Design review of the part built by this model. Coordinates are the model's own, in mm. A direction names the side the tool comes from. Coordinates: 2 decimals unless noted, no trailing zeros. Write each loop counter-clockwise with the first axis right and the second up, starting at its lowest first coordinate (ties: lowest second). Pieces come first, ordered by that corner, then holes. Notation, with made-up numbers: (-20, 13.25) - (16, 13.25) arc R31 cw to (16, 52.25) - close; hole circle Ø6 at (75.5, 65.25). An arc over 180 degrees is marked (long way). Answer as a JSON object with one key per item and string values.
```python
from build123d import *

# Parameters (mm, degrees)
SKETCH2_W               = 52
SKETCH2_H               = 58.5
SKETCH2_R               = 1.7
SKETCH2_R_2             = 2.65
BOSS_EXTRUDE1_DEPTH     = 5
SKETCH2_3_R             = 2.65
SKETCH2_3_R_2           = 1.5
BOSS_EXTRUDE2_DEPTH     = 2
SKETCH3_R               = 3
SKETCH3_R_2             = 1.7
BOSS_EXTRUDE3_DEPTH     = 6.5
CUT_EXTRUDE1_DEPTH      = 45.082309377
CUT_EXTRUDE1_DEPTH_BACK = 45.082309377
SKETCH4_R               = 4.5
SKETCH4_R_2             = 3.2
FILLET1_R               = 2.5


with BuildPart() as part:
    # Sketch2 → Boss-Extrude1 (new body)
    with BuildSketch(Plane.XY):
        with Locations((0, -5.75)):
            Rectangle(SKETCH2_W, SKETCH2_H)
        with Locations((-20, -23)):
            Circle(SKETCH2_R, mode=Mode.SUBTRACT)
        with Locations((20, -23)):
            Circle(SKETCH2_R, mode=Mode.SUBTRACT)
        with Locations((20, 15)):
            Circle(SKETCH2_R, mode=Mode.SUBTRACT)
        with Locations((-20, 15)):
            Circle(SKETCH2_R, mode=Mode.SUBTRACT)
        with Locations((-17.5, 0)):
            Circle(SKETCH2_R_2, mode=Mode.SUBTRACT)
        with Locations((0, -17.5)):
            Circle(SKETCH2_R_2, mode=Mode.SUBTRACT)
        with Locations((17.5, 0)):
            Circle(SKETCH2_R_2, mode=Mode.SUBTRACT)
        with Locations((0, 17.5)):
            Circle(SKETCH2_R_2, mode=Mode.SUBTRACT)
    extrude(amount=BOSS_EXTRUDE1_DEPTH)

    # Sketch2_3 → Boss-Extrude2 (add)
    # profile 1 of 4: a face of its own
    with BuildSketch(Plane.XY):
        with Locations((0, 17.5)):
            Circle(SKETCH2_3_R)
        with Locations((0, 17.5)):
            Circle(SKETCH2_3_R_2, mode=Mode.SUBTRACT)
    # profile 2 of 4: a face of its own
    with BuildSketch(Plane.XY):
        with Locations((-17.5, 0)):
            Circle(SKETCH2_3_R)
        with Locations((-17.5, 0)):
            Circle(SKETCH2_3_R_2, mode=Mode.SUBTRACT)
    # profile 3 of 4: a face of its own
    with BuildSketch(Plane.XY):
        with Locations((17.5, 0)):
            Circle(SKETCH2_3_R)
        with Locations((17.5, 0)):
            Circle(SKETCH2_3_R_2, mode=Mode.SUBTRACT)
    # profile 4 of 4: a face of its own
    with BuildSketch(Plane.XY):
        with Locations((0, -17.5)):
            Circle(SKETCH2_3_R)
        with Locations((0, -17.5)):
            Circle(SKETCH2_3_R_2, mode=Mode.SUBTRACT)
    extrude(amount=BOSS_EXTRUDE2_DEPTH)

    # Sketch3 → Boss-Extrude3 (add)
    # profile 1 of 4: a face of its own
    with BuildSketch(Plane.XY.offset(5)):
        with Locations(Location((-20, 15, 0), (0, 0, 180))):
            Circle(SKETCH3_R)
        with Locations((-20, 15)):
            Circle(SKETCH3_R_2, mode=Mode.SUBTRACT)
    # profile 2 of 4: a face of its own
    with BuildSketch(Plane.XY.offset(5)):
        with Locations(Location((20, 15, 0), (0, 0, 180))):
            Circle(SKETCH3_R)
        with Locations((20, 15)):
            Circle(SKETCH3_R_2, mode=Mode.SUBTRACT)
    # profile 3 of 4: a face of its own
    with BuildSketch(Plane.XY.offset(5)):
        with Locations(Location((-20, -23, 0), (0, 0, 180))):
            Circle(SKETCH3_R)
        with Locations((-20, -23)):
            Circle(SKETCH3_R_2, mode=Mode.SUBTRACT)
    # profile 4 of 4: a face of its own
    with BuildSketch(Plane.XY.offset(5)):
        with Locations(Location((20, -23, 0), (0, 0, 180))):
            Circle(SKETCH3_R)
        with Locations((20, -23)):
            Circle(SKETCH3_R_2, mode=Mode.SUBTRACT)
    extrude(amount=BOSS_EXTRUDE3_DEPTH)

    # Sketch4 → Cut-Extrude1 (cut, two sides: drawn at the far end of the back side and taken through both)
    # profile 1 of 2: a face of its own
    with BuildSketch(Plane.XY.offset(5).offset(-CUT_EXTRUDE1_DEPTH_BACK)):
        Circle(SKETCH4_R)
        Circle(SKETCH4_R_2, mode=Mode.SUBTRACT)
    # profile 2 of 2: a face of its own
    with BuildSketch(Plane.XY.offset(5).offset(-CUT_EXTRUDE1_DEPTH_BACK)):
        Circle(SKETCH4_R_2)
    extrude(amount=CUT_EXTRUDE1_DEPTH + CUT_EXTRUDE1_DEPTH_BACK, mode=Mode.SUBTRACT)

    # Fillet1
    fillet1_edges = [part.edges().sort_by_distance(p)[0] for p in [
        (-17, 15, 5),
        (23, 15, 5),
        (-17, -23, 5),
        (23, -23, 5),
    ]]
    fillet(fillet1_edges, radius=FILLET1_R)


solid = part.part
```
(1) For pin 1 (1.6 mm diameter, centred on x = 1, y = -17.5, fed in from +Z); pin 2 (1 mm diameter, centred on x = 1.5, y = -11, fed in from +Z); pin 3 (5 mm diameter, centred on y = -21.5, z = 8.5, fed in from +X), all flat-tipped, find the tip position at first contact; note any pin that passes through.
Solved:
{"pin 1": "stops at z = 2", "pin 2": "stops at z = 5", "pin 3": "stops at x = 23.34"}
(2) Take a section at A-A, the plane z = 9.5. Write out the cut boundary in (x, y).
Solved:
{"outline": "circle Ø6 at (-20, -23); circle Ø6 at (-20, 15); circle Ø6 at (20, -23); circle Ø6 at (20, 15); hole circle Ø3.4 at (-20, -23); hole circle Ø3.4 at (-20, 15); hole circle Ø3.4 at (20, -23); hole circle Ø3.4 at (20, 15)"}
(3) Take a section at D-D, the plane z = 3.5. Give the number of separate pieces and of enclosed holes in the cut face, and give its area (3 significant figures).
Solved:
{"separate pieces": "1", "enclosed holes": "9", "area": "2,850 mm^2"}
(4) Take a section at B-B, the plane y = -23. Write out the cut boundary in (x, z), and give its area (3 significant figures).
Solved:
{"outline": "(-26, 0) - (-21.7, 0) - (-21.7, 11.5) - (-23, 11.5) - (-23, 7.5) arc R2.5 cw to (-25.5, 5) - (-26, 5) - close; (-18.3, 0) - (18.3, 0) - (18.3, 11.5) - (17, 11.5) - (17, 7.5) arc R2.5 cw to (14.5, 5) - (-14.5, 5) arc R2.5 cw to (-17, 7.5) - (-17, 11.5) - (-18.3, 11.5) - close; (21.7, 0) - (26, 0) - (26, 5) - (25.5, 5) arc R2.5 cw to (23, 7.5) - (23, 11.5) - (21.7, 11.5) - close", "area": "265 mm^2"}
(5) Take a section at C-C, the plane x = 0. Write out the cut boundary in (y, z).
Solved:
{"outline": "(-35, 0) - (-19, 0) - (-19, 2) - (-20.15, 2) - (-20.15, 5) - (-35, 5) - close; (-16, 0) - (-4.5, 0) - (-4.5, 5) - (-14.85, 5) - (-14.85, 2) - (-16, 2) - close; (4.5, 0) - (16, 0) - (16, 2) - (14.85, 2) - (14.85, 5) - (4.5, 5) - close; (19, 0) - (23.5, 0) - (23.5, 5) - (20.15, 5) - (20.15, 2) - (19, 2) - close"}
(6) The part is to be moulded in two halves that separate along Y. For faces 1 (the face through (18, -23, 11.5)), 2 (the face through (-0.34, 20.13, 3.48)), 3 (the face through (0, -35, 2)), say which applies: pulls with the +Y half, pulls with the -Y half, needs draft (parallel to the pull), parting line crosses it, or undercut.
Solved:
{"face 1": "needs draft", "face 2": "undercut", "face 3": "pulls with the -Y half"}
(7) To check wall thickness, follow line 1 (Y direction, x = 0, z = 3.8); line 2 (Y direction, x = 20, z = 7.5); line 3 (Y direction, x = 17.5, z = 2.85). State the ranges of each line that lie inside material, in increasing order. Write a range as from..to.
Solved:
{"line 1": "y = -35..-20.15, -14.85..-4.5, 4.5..14.85, 20.15..23.5", "line 2": "y = -26..-24.7, -21.3..-20, 12..13.3, 16.7..18", "line 3": "y = -35..-2.65, 2.65..23.5"}
(8) Tool access review of faces 4 (the face through (1.223, -19.851, 3.479)), 5 (the face through (20, 17, 11.5)): name each direction out of +Z, -Z, +X, -X, +Y, -Y from which nothing blocks a thin tool from reaching the whole face with its end or side.
Solved:
{"face 4": "+Z", "face 5": "+Z, +X, -X, +Y, -Y"}
